Build history of the part. All positions in model axes, mm. A direction names the side the tool comes from. Give positions to 0.01 mm unless a question says otherwise; leave off trailing zeros. Loops run counter-clockwise (first coordinate to the right, second up) from the corner with the lowest first, then second, coordinate; pieces in that order, holes last. Notation, with made-up numbers: (63.5, 22.25) -> (103.5, 22.25) arc R6 cw to (103.5, 30.25) -> close; hole circle Ø6 at (62.5, -34.75). An arc over 180 degrees is marked (long way). Answer as a JSON object with one key per item and string values. Group by question number.
Q1. Band-saw the part on A-A, the plane y = 0. Write the cut outline in (x, z).
Q2. Tool access for faces 5 (the cylindrical face through (4.1, -9.14, 3.94)), 6 (the flat face through (-2.028, -3.448, 6.028)): list every direction of +Z, -Z, +X, -X, +Y, -Y with a clear straight run to the whole face (end or side of a thin tool).
Q3. Two-plate mould, pull along X, no slides. Class faces 1 (the cylindrical face through (4.14, 9.1, 3.94)), 2 (the flat face through (4, 0, 6)), 3 (the cylindrical face through (-4.14, -9.1, 3.94)), 4 (the flat face through (-1.2, 2.4, 0)): pulls with the +X half, pulls with the -X half, needs draft (parallel to the pull), parting line crosses it, or undercut.
Q4. Band-saw the part on B-B, the plane x = 0.75. Write the cut outline in (y, z).
Q5. Wall check: probe 1 along Y at (x, z) = (0, 1.55); probe 2 along X at (y, z) = (1.25, 5.5); probe 3 along Z at (x, y) = (2.5, -0.75). Give the ranges that are in metal, low to high. Write a range as from..to.
Q6. Band-saw the part on C-C, the plane z = 5.75. Write the cut outline in (x, y).
Q7. Band-saw the part on D-D, the plane x = 2.75. Write the cut outline in (y, z), plus the area to 3 significant figures.
Q8. Drop a flat-ended pin along its axis: pin 1 (1 mm diameter, centred on x = -3, z = 2, fed in from -Y). Give the stop position or say it passes through.
from build123d import *

# Parameters (mm, degrees)
F1_DEPTH = 8
F2_R     = 2.5
F3_DEPTH = 25
F5_DEPTH = 4


with BuildPart() as f1:
    # F0 (on Top) → F1 (new body)
    with BuildSketch(Plane.XY):
        with BuildLine():
            Line((-2, -10), (2, -10))
            ThreePointArc((2, -10), (4.12132, -9.12132), (5, -7))
            Line((5, -7), (5, 7))
            ThreePointArc((5, 7), (4.12132, 9.12132), (2, 10))
            Line((2, 10), (-2, 10))
            ThreePointArc((-2, 10), (-4.12132, 9.12132), (-5, 7))
            Line((-5, 7), (-5, -7))
            ThreePointArc((-5, -7), (-4.12132, -9.12132), (-2, -10))
        make_face()
    extrude(amount=F1_DEPTH)

    # F2 (on face) → F3 (cut)
    with BuildSketch(Plane.XY.offset(8)):
        Circle(F2_R)
    extrude(amount=-F3_DEPTH, mode=Mode.SUBTRACT)

    # F4 (on face) → F5 (cut)
    with BuildSketch(Plane.XY.offset(8)):
        Polygon((0, -4.618802), (4, -2.309401), (4, 2.309401), (0, 4.618802), (-4, 2.309401), (-4, -2.309401), align=None)
    extrude(amount=-F5_DEPTH, mode=Mode.SUBTRACT)


solid = f1.part
Worked answers:
{
 "1": {"outline": "(-5, 0) -> (-2.5, 0) -> (-2.5, 4) -> (-4, 4) -> (-4, 8) -> (-5, 8) -> close; (2.5, 0) -> (5, 0) -> (5, 8) -> (4, 8) -> (4, 4) -> (2.5, 4) -> close"},
 "2": {"face 5": "+Z, -Z, +X, -Y", "face 6": "+Z"},
 "3": {"face 1": "pulls with the +X half", "face 2": "undercut", "face 3": "pulls with the -X half", "face 4": "needs draft"},
 "4": {"outline": "(-10, 0) -> (-2.38, 0) -> (-2.38, 4) -> (-4.19, 4) -> (-4.19, 8) -> (-10, 8) -> close; (2.38, 0) -> (10, 0) -> (10, 8) -> (4.19, 8) -> (4.19, 4) -> (2.38, 4) -> close"},
 "5": {"probe 1": "-10..-2.5, 2.5..10", "probe 2": "-5..-4, 4..5", "probe 3": "0..4"},
 "6": {"outline": "(-5, -7) arc R3 ccw to (-2, -10) -> (2, -10) arc R3 ccw to (5, -7) -> (5, 7) arc R3 ccw to (2, 10) -> (-2, 10) arc R3 ccw to (-5, 7) -> close; hole (-4, -2.31) -> (0, -4.62) -> (4, -2.31) -> (4, 2.31) -> (0, 4.62) -> (-4, 2.31) -> close"},
 "7": {"outline": "(-9.9, 0) -> (9.9, 0) -> (9.9, 8) -> (3.03, 8) -> (3.03, 4) -> (-3.03, 4) -> (-3.03, 8) -> (-9.9, 8) -> close", "area": "134 mm2"},
 "8": {"pin 1": "y = -9.96"}
}
